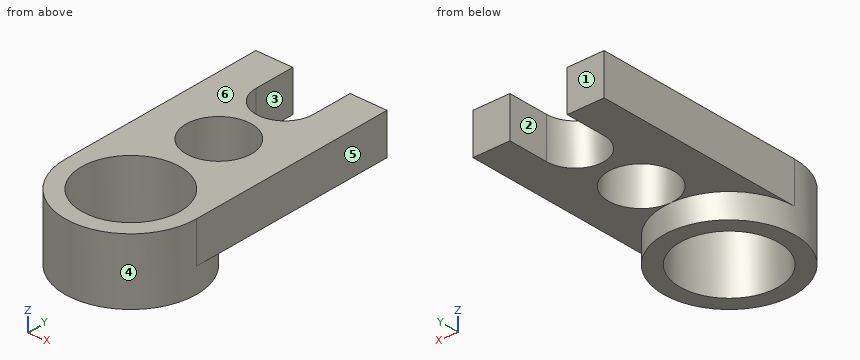
from build123d import *

# Parameters (mm, degrees)
ESQUISSE1_R          = 4
BASE_EXTRUSION_DEPTH = 5
BOSS_EXTRU_1_START   = -8
ESQUISSE2_R          = 8
BOSS_EXTRU_1_DEPTH   = 8
PER_AGE1_D           = 12
PER_AGE1_DEPTH       = 8
PER_AGE1_TIP         = 3.605163714


with BuildPart() as part:
    # Esquisse1 → Base-Extrusion (new body)
    with BuildSketch(Plane.XY):
        with BuildLine():
            Line((-25.742801556, 26), (-30.242801556, 26))
            Line((-30.242801556, 26), (-30.242801556, 0))
            ThreePointArc((-30.242801556, 0), (-22.242801556, -8), (-14.242801556, 0))
            Line((-14.242801556, 0), (-14.242801556, 26))
            Line((-14.242801556, 26), (-18.742801556, 26))
            Line((-18.742801556, 26), (-18.742801556, 21))
            ThreePointArc((-18.742801556, 21), (-22.242801556, 17.5), (-25.742801556, 21))
            Line((-25.742801556, 21), (-25.742801556, 26))
        make_face()
        with Locations(Location((-22.242801556, 12, 0), (0, 0, 270))):
            Circle(ESQUISSE1_R, mode=Mode.SUBTRACT)
    extrude(amount=BASE_EXTRUSION_DEPTH)

    # Esquisse2 → Boss.-Extru.1 (add)
    with BuildSketch(Plane.XY.offset(5).offset(BOSS_EXTRU_1_START)):
        with Locations((-22.242801556, 0)):
            Circle(ESQUISSE2_R)
    extrude(amount=BOSS_EXTRU_1_DEPTH)

    # Perçage1
    with Locations(Plane(origin=(0, 0, -3), x_dir=(-1, 0, 0), z_dir=(0, 0, -1))):
        with Locations((22.242801556, 0)):
            Hole(PER_AGE1_D / 2, depth=PER_AGE1_DEPTH)
            with Locations((0, 0, -(PER_AGE1_DEPTH + PER_AGE1_TIP / 2))):  # 118° drill point
                Cone(0, PER_AGE1_D / 2, PER_AGE1_TIP, mode=Mode.SUBTRACT)


solid = part.part
Can you work these out from the model? Positions are in its coordinate system, mm. Face numbers are marked on the shaded views. A direction names the side the tool comes from. Give positions to 0.01 mm unless a question says otherwise; leave off trailing zeros. Loops run counter-clockwise (first coordinate to the right, second up) from the corner with the lowest first, then second, coordinate; pieces in that order, holes last. Notation, with made-up numbers: (7, 17.25) -> (14, 17.25) arc R23 ccw to (14, 27.25) -> close; hole circle Ø11 at (14, 24.5). An arc over 180 degrees is marked (long way). Write item = value, one per line.
1) Suppose I cut it at A-A on y = 12. Write out the boundary of the cut face in (x, z).
Check result:
outline = (-30.24, 0) -> (-26.24, 0) -> (-26.24, 5) -> (-30.24, 5) -> close; (-18.24, 0) -> (-14.24, 0) -> (-14.24, 5) -> (-18.24, 5) -> close
2) Will these pins go through, and if not, where does the flat tip stop? pin 1 (5 mm diameter, centred on x = -22.24, y = 12, fed in from +Z); pin 2 (1.5 mm diameter, centred on x = -28.5, y = 20.5, fed in from -Z); pin 3 (5 mm diameter, centred on x = -17.5, y = 2.5, fed in from -Z); pin 4 (1.5 mm diameter, centred on x = -28, z = -0.5, fed in from -Y).
Check result:
pin_1 = through
pin_2 = 0
pin_3 = -3
pin_4 = -6.24
3) Suppose I cut it at B-B on x = -20.5. Write out the boundary of the cut face in (y, z), then the cut area to 3 significant figures.
Check result:
outline = (-7.81, -3) -> (-5.74, -3) -> (-5.74, 5) -> (-7.81, 5) -> close; (5.74, -3) -> (7.81, -3) -> (7.81, 0) -> (8.4, 0) -> (8.4, 5) -> (5.74, 5) -> close; (15.6, 0) -> (17.96, 0) -> (17.96, 5) -> (15.6, 5) -> close
area = 47.8 mm2
4) For the marked faces 1 and 2, which set-ups out of +Z, -Z, +X, -X, +Y, -Y let a thin tool reach every point of the face, with its end or its side?
Check result:
face_1 = +Z, -Z, +X, -X, +Y
face_2 = +Z, -Z, +Y
5) I need wall thicknesses on L1, parallel to Y at x = -22, z = 3; L2, parallel to X at y = 0, z = -1.5; L3, parallel to Y at x = -24.25, z = 4.75. Which ranges of each line are inside material? Lowest first, please. Write a range as from..to.
Check result:
L1 = -8..-6, 6..8.01, 15.99..17.51
L2 = -30.24..-28.24, -16.24..-14.24
L3 = -7.74..-5.65, 5.65..8.54, 15.46..18.13
6) Suppose I cut it at D-D on y = -2. Write out the boundary of the cut face in (x, z).
Check result:
outline = (-29.99, -3) -> (-27.9, -3) -> (-27.9, 5) -> (-29.99, 5) -> close; (-16.59, -3) -> (-14.5, -3) -> (-14.5, 5) -> (-16.59, 5) -> close
7) Suppose I cut it at C-C on z = -1.5. Write out the boundary of the cut face in (x, y), then the cut area to 3 significant figures.
Check result:
outline = circle Ø16 at (-22.24, 0); hole circle Ø12 at (-22.24, 0)
area = 88.0 mm2
8) Thinking about a two-plate mould opening in X: for the marked faces 3, 4, 5 and 6, which applies, released by +X, released by -X, zero draft, split by the parting line, or undercut?
Check result:
face_3 = undercut
face_4 = split by the parting line
face_5 = released by +X
face_6 = zero draft
